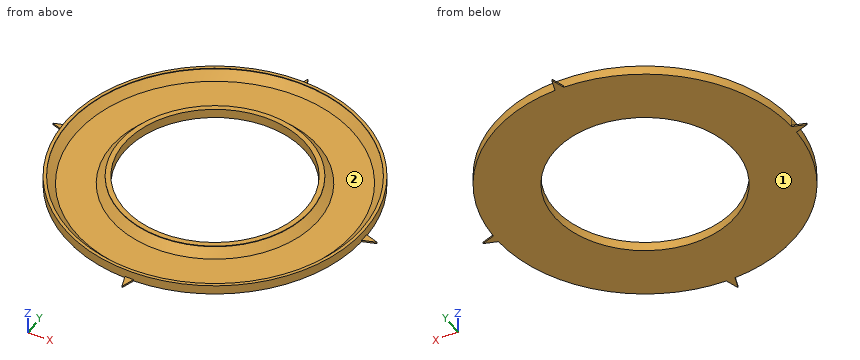
```python
from build123d import *

# Parameters (mm, degrees)
F0_R            = 95
F0_R_2          = 62
F0_R_3          = 58.75
F1_DEPTH        = 0.6
F2_DEPTH        = 6
F3_DEPTH        = 1
F3_COPIES_COUNT = 4
F4_SIZE         = 5


# Not quite as in the source:
# - a pattern or mirror of a feature is missing from the dataset's text; its kind, count and spacing are read off the source's solid


with BuildPart() as f1:
    # F0 (on Top) → F1 (new body)
    with BuildSketch(Plane.XY):
        with BuildLine():
            ThreePointArc((-96.9585308057, -2.8360719318), (1.418187549, -96.9896321473), (97, 0))
            ThreePointArc((97, 0), (1.418187549, 96.9896321473), (-96.9585308057, 2.8360719318))
            ThreePointArc((-96.9585308057, 2.8360719318), (-96.9896321473, 1.418187549), (-97, 0))
            ThreePointArc((-97, 0), (-96.9896321473, -1.418187549), (-96.9585308057, -2.8360719318))
        make_face()
        Circle(F0_R, mode=Mode.SUBTRACT)
        Circle(F0_R)
        Circle(F0_R_2, mode=Mode.SUBTRACT)
        Circle(F0_R_2)
        Circle(F0_R_3, mode=Mode.SUBTRACT)
    extrude(amount=F1_DEPTH)

    # F0 (on Top) → F2 (join)
    with BuildSketch(Plane.XY):
        with BuildLine():
            ThreePointArc((-96.9585308057, -2.8360719318), (1.418187549, -96.9896321473), (97, 0))
            ThreePointArc((97, 0), (1.418187549, 96.9896321473), (-96.9585308057, 2.8360719318))
            ThreePointArc((-96.9585308057, 2.8360719318), (-96.9896321473, 1.418187549), (-97, 0))
            ThreePointArc((-97, 0), (-96.9896321473, -1.418187549), (-96.9585308057, -2.8360719318))
        make_face()
        Circle(F0_R, mode=Mode.SUBTRACT)
        Circle(F0_R_2)
        Circle(F0_R_3, mode=Mode.SUBTRACT)
    extrude(amount=F2_DEPTH)

    # F0 (on Top) → F3 (join)
    with BuildSketch(Plane.XY):
        with BuildLine():
            ThreePointArc((-97, 0), (-96.9896321473, 1.418187549), (-96.9585308057, 2.8360719318))
            Line((-96.9585308057, 2.8360719318), (-105.5, 0))
            Line((-105.5, 0), (-97, 0))
        make_face()
        with BuildLine():
            Line((-105.5, 0), (-96.9585308057, -2.8360719318))
            ThreePointArc((-96.9585308057, -2.8360719318), (-96.9896321473, -1.418187549), (-97, 0))
            Line((-97, 0), (-105.5, 0))
        make_face()
    f3 = extrude(amount=F3_DEPTH)

    # F3_copies: F3 ×4 about axis
    f3_copies_axis = Axis((0, 0, 0), (0, 0, 1))
    for i in range(1, F3_COPIES_COUNT):
        add(f3.rotate(f3_copies_axis, i * 360 / F3_COPIES_COUNT))

    # F4
    f4_edges = [f1.edges().sort_by_distance(p)[0] for p in [
        (-62, 0, 0.6),
        (-95, 0, 0.6),
    ]]
    chamfer(f4_edges, length=F4_SIZE)


solid = f1.part
```
Read the model definition and answer for the solid it produces. Units are mm, in the model's axes. Face numbers are marked on the shaded views. Coordinates: 2 decimals unless noted, no trailing zeros. Order: outer loops, then holes, each group sorted by start corner. A loop starts at its lowest first (then second) coordinate and runs counter-clockwise, first axis right, second up. Notation, with made-up numbers: (56, -34) - (69, -34) arc R23 cw to (69, 0) - close; hole circle Ø7 at (-27.5, -22.75). An arc over 180 degrees is marked (long way). Answer as a JSON object with one key per item and string values. Group by question number.
Item 1: Flat-ended cylindrical pins translate along their axes: P1, Ø3, axis at x = -64.5, y = 56.5, coming from the +Z side; P2, Ø3, axis at x = -35, z = 2, coming from the +Y side; P3, Ø1.7, axis at x = 103, y = -1.5, coming from the +Z side. Find the tip coordinate at first contact, or state that the pin passes through.
Item 2: The mould has two halves that part along X. Classify the marked faces 1 and 2: +X half, -X half, draft (parallel to the pull), parting line (faces both ways), or undercut.
Item 3: Consider probe 1 along Y at (x, z) = (0, 5.9); probe 2 along Y at (x, z) = (8, 3.3); probe 3 along X at (y, z) = (-46, 5.2). Determine where each line is inside the solid, lowest interval first. Write a range as from..to.
Item 4: Section A-A (z = 2.45) is taken. Give the vertices of the cut face in (x, y), plus the area to 3 significant figures.
Results are:
{
 "1": {"P1": "stops at z = 0.6", "P2": "stops at y = 91.03", "P3": "stops at z = 1"},
 "2": {"face 1": "draft", "face 2": "undercut"},
 "3": {"probe 1": "y = -97..-95, -62..-58.75, 58.75..62, 95..97", "probe 2": "y = -96.67..-92.35, -63.8..-58.2, 58.2..63.8, 92.35..96.67", "probe 3": "x = -85.4..-82.66, -42.16..-36.55, 36.55..42.16, 82.66..85.4"},
 "4": {"outline": "circle Ø194 at (0, 0); circle Ø130.3 at (0, 0); hole circle Ø183.7 at (0, 0); hole circle Ø117.5 at (0, 0)", "area": "5,550 mm^2"}
}
